Part print with two shaded views. Sizes in mm from the minimum x, y, z corner. Coordinates: 2 decimals unless noted, no trailing zeros. Order: outer loops, then holes, each group sorted by start corner. A loop starts at its lowest first (then second) coordinate and runs counter-clockwise, first axis right, second up.
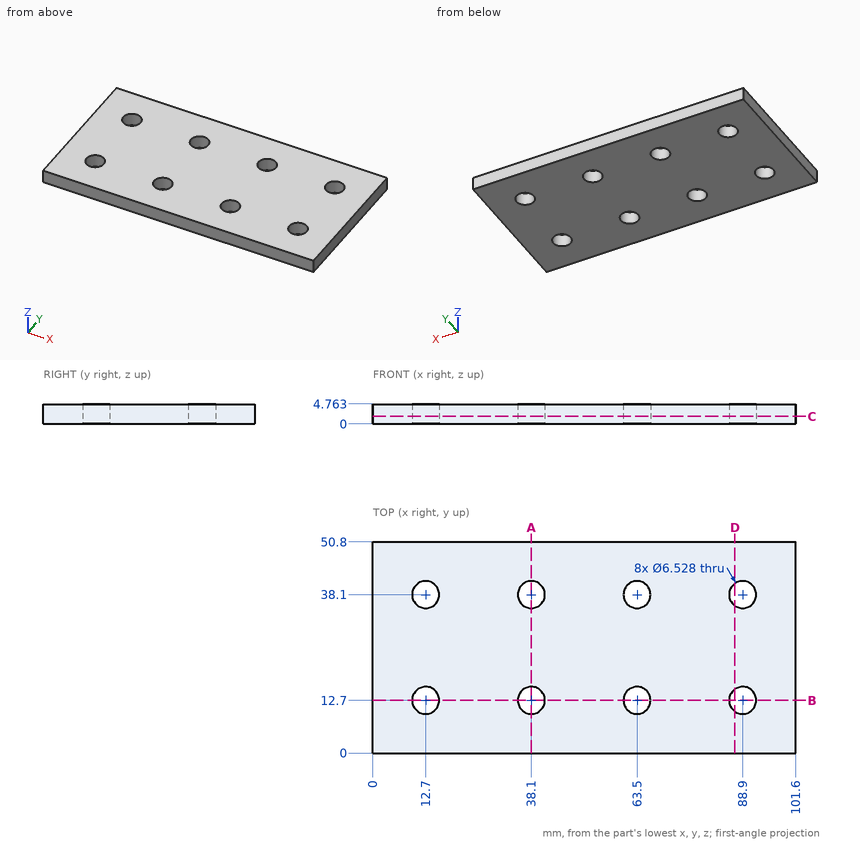
Q1. Wall check: line 1 along X through (y, z) = (38.1, 1.4); line 2 along Y through (x, z) = (63.5, 2.85); line 3 along X through (y, z) = (37, 4). Give the ranges that are in metal, low to high.
Results list:
line 1: x = 0 to 9.44, 15.96 to 34.84, 41.36 to 60.24, 66.76 to 85.64, 92.16 to 101.6
line 2: y = 0 to 9.44, 15.96 to 34.84, 41.36 to 50.8
line 3: x = 0 to 9.63, 15.77 to 35.03, 41.17 to 60.43, 66.57 to 85.83, 91.97 to 101.6
Q2. Cut at B-B on y = 12.7. Write the cut outline in (x, z).
Results list:
outline: (0, 0) - (9.44, 0) - (9.44, 4.76) - (0, 4.76) - close; (15.96, 0) - (34.84, 0) - (34.84, 4.76) - (15.96, 4.76) - close; (41.36, 0) - (60.24, 0) - (60.24, 4.76) - (41.36, 4.76) - close; (66.76, 0) - (85.64, 0) - (85.64, 4.76) - (66.76, 4.76) - close; (92.16, 0) - (101.6, 0) - (101.6, 4.76) - (92.16, 4.76) - close
Q3. Cut at A-A on x = 38.1. Write the cut outline in (y, z), and give its area (3 significant figures).
Results list:
outline: (0, 0) - (9.44, 0) - (9.44, 4.76) - (0, 4.76) - close; (15.96, 0) - (34.84, 0) - (34.84, 4.76) - (15.96, 4.76) - close; (41.36, 0) - (50.8, 0) - (50.8, 4.76) - (41.36, 4.76) - close
area: 180 mm2
Q4. Cut at D-D on x = 87. Write the cut outline in (y, z).
Results list:
outline: (0, 0) - (10.05, 0) - (10.05, 4.76) - (0, 4.76) - close; (15.35, 0) - (35.45, 0) - (35.45, 4.76) - (15.35, 4.76) - close; (40.75, 0) - (50.8, 0) - (50.8, 4.76) - (40.75, 4.76) - close
Q5. Cut at C-C on z = 1.8. Count the separate pieces of the cut face and the enclosed holes in it, and give its area (3 significant figures).
Results list:
separate pieces: 1
enclosed holes: 8
area: 4,890 mm2
